from build123d import *

# Parameters (mm, degrees)
F0_W     = 2000
F0_H     = 1750
F0_W_2   = 952
F0_H_2   = 32
F0_W_3   = 32
F0_H_3   = 827
F0_W_4   = 356
F1_DEPTH = 32


# Not quite as in the source:
# - a feature names something its author has since deleted; it is built from what else it names


with BuildPart() as f1:
    # F0 (on Front) → F1 (new body)
    with BuildSketch(Plane.XZ):
        with Locations((1000, 875)):
            Rectangle(F0_W, F0_H)
        Polygon((984, 32), (32, 32), (32, 859), (32, 891), (32, 1718), (984, 1718), (1016, 1718), (1968, 1718), (1968, 1564), (1968, 1532), (1968, 891), (1968, 859), (1968, 32), (1404, 32), (1372, 32), (1016, 32), align=None, mode=Mode.SUBTRACT)
        with Locations((508, 875)):
            Rectangle(F0_W_2, F0_H_2)
        with Locations((1000, 445.5)):
            Rectangle(F0_W_3, F0_H_3)
        with Locations((1000, 875)):
            Rectangle(F0_W_3, F0_H_2)
        Polygon((984, 1718), (984, 891), (1016, 891), (1016, 1532), (1016, 1564), (1016, 1718), align=None)
        with Locations((1194, 875)):
            Rectangle(F0_W_4, F0_H_2)
        Polygon((1372, 859), (1372, 32), (1404, 32), (1404, 1532), (1372, 1532), (1372, 891), align=None)
        Polygon((1016, 1564), (1016, 1532), (1372, 1532), (1404, 1532), (1968, 1532), (1968, 1564), align=None)
    extrude(amount=F1_DEPTH)


solid = f1.part
For this review, take the finished solid that the model builds, in its own axes (mm). Round coordinates to 2 decimals unless told otherwise and drop trailing zeros. Write each loop counter-clockwise with the first axis right and the second up, starting at its lowest first coordinate (ties: lowest second). Pieces come first, ordered by that corner, then holes. Notation, with made-up numbers: (-21, 46) - (16, 46) arc R21 ccw to (16, 75) - close; hole circle Ø9 at (79, 44.5). An arc over 180 degrees is marked (long way). Use a Markdown table: item, result.
Q1. We need section C-C (z = 1370). Give the boundary of the cut face in (x, y).
Derived:
| item | result |
|---|---|
| outline | (0, -32) - (32, -32) - (32, 0) - (0, 0) - close; (984, -32) - (1016, -32) - (1016, 0) - (984, 0) - close; (1372, -32) - (1404, -32) - (1404, 0) - (1372, 0) - close; (1968, -32) - (2000, -32) - (2000, 0) - (1968, 0) - close |
Q2. Wall thickness on line 1 along Z through (x, y) = (275, -5); line 2 along X through (y, z) = (-22.5, 1217); line 3 along Z through (x, y) = (1529, -8.5): over which ranges is each line inside the solid? List them lowest first.
Derived:
| item | result |
|---|---|
| line 1 | z = 0 to 32, 859 to 891, 1718 to 1750 |
| line 2 | x = 0 to 32, 984 to 1016, 1372 to 1404, 1968 to 2000 |
| line 3 | z = 0 to 32, 1532 to 1564, 1718 to 1750 |
Q3. We need section A-A (x = 1232.5). Give the boundary of the cut face in (y, z), plus the area to 3 significant figures.
Derived:
| item | result |
|---|---|
| outline | (-32, 0) - (0, 0) - (0, 32) - (-32, 32) - close; (-32, 859) - (0, 859) - (0, 891) - (-32, 891) - close; (-32, 1532) - (0, 1532) - (0, 1564) - (-32, 1564) - close; (-32, 1718) - (0, 1718) - (0, 1750) - (-32, 1750) - close |
| area | 4,100 mm2 |
Q4. We need section D-D (x = 1698). Give the boundary of the cut face in (y, z), plus the area to 3 significant figures.
Derived:
| item | result |
|---|---|
| outline | (-32, 0) - (0, 0) - (0, 32) - (-32, 32) - close; (-32, 1532) - (0, 1532) - (0, 1564) - (-32, 1564) - close; (-32, 1718) - (0, 1718) - (0, 1750) - (-32, 1750) - close |
| area | 3,070 mm2 |
Q5. We need section B-B (y = -11). Give the boundary of the cut face in (x, z), plus the area to 3 significant figures.
Derived:
| item | result |
|---|---|
| outline | (0, 0) - (2000, 0) - (2000, 1750) - (0, 1750) - close; hole (32, 32) - (984, 32) - (984, 859) - (32, 859) - close; hole (32, 891) - (984, 891) - (984, 1718) - (32, 1718) - close; hole (1016, 32) - (1372, 32) - (1372, 859) - (1016, 859) - close; hole (1016, 891) - (1372, 891) - (1372, 1532) - (1016, 1532) - close; hole (1016, 1564) - (1968, 1564) - (1968, 1718) - (1016, 1718) - close; hole (1404, 32) - (1968, 32) - (1968, 1532) - (1404, 1532) - close |
| area | 410,000 mm2 |
